Geometry check sheet. Reference: the model listing, model coordinates, mm. Face numbers are marked on the shaded views. A direction names the side the tool comes from. Round coordinates to 2 decimals unless told otherwise and drop trailing zeros. Loops run counter-clockwise (first coordinate to the right, second up) from the corner with the lowest first, then second, coordinate; pieces in that order, holes last.
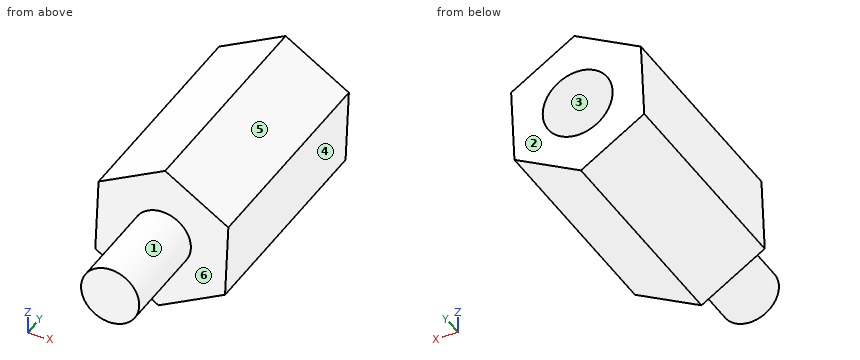
```python
from build123d import *

# Parameters (mm, degrees)
BOSS_EXTRUDE1_DEPTH = 11.1125
SKETCH2_R           = 1.4224
BOSS_EXTRUDE2_DEPTH = 4.7625
SKETCH3_R           = 1.70891155
CUT_EXTRUDE1_DEPTH  = 6.35


with BuildPart() as part:
    # Sketch1 → Boss-Extrude1 (new body)
    with BuildSketch(Plane(origin=(0, 0, 0), x_dir=(1, 0, 0), z_dir=(0, 1, 0))):
        Polygon((3.252691355, -1.691399504), (3.091140616, 1.971213592), (-0.161550739, 3.662613096), (-3.252691355, 1.691399504), (-3.091140616, -1.971213592), (0.161550739, -3.662613096), align=None)
    extrude(amount=BOSS_EXTRUDE1_DEPTH)

    # Sketch2 → Boss-Extrude2 (add)
    with BuildSketch(Plane.XZ):
        Circle(SKETCH2_R)
    extrude(amount=BOSS_EXTRUDE2_DEPTH)

    # Sketch3 → Cut-Extrude1 (cut)
    with BuildSketch(Plane(origin=(0, 11.1125, 0), x_dir=(1, 0, 0), z_dir=(0, 1, 0))):
        Circle(SKETCH3_R)
    extrude(amount=-CUT_EXTRUDE1_DEPTH, mode=Mode.SUBTRACT)


solid = part.part
```
1) Mould release check, pull along Z, two halves, no side actions. Record for the marked faces 3, 4, 5 and 6: +Z half, -Z half, draft (parallel to the pull), parting line (faces both ways), or undercut.
Report:
face 3: undercut
face 4: -Z half
face 5: +Z half
face 6: draft
2) Gauge pin test, flat ends, axial feed: pin 1 (1 mm diameter, centred on x = -1.5, y = 2, fed in from +Z); pin 2 (4 mm diameter, centred on y = 0.5, z = 0.5, fed in from -X); pin 3 (1.5 mm diameter, centred on y = 2.5, z = 0.5, fed in from +X). Record the tip position at first contact, or that the pin passes through.
Report:
pin 1: stops at z = 3.06
pin 2: stops at x = -3.24
pin 3: stops at x = 3.23
3) Sectioned sample at A-A, the plane y = 6. Record the cut outline in (x, z), then the cut area to 3 significant figures.
Report:
outline: (-3.25, -1.69) - (-0.16, -3.66) - (3.09, -1.97) - (3.25, 1.69) - (0.16, 3.66) - (-3.09, 1.97) - close; hole circle Ø3.42 at (0, 0)
area: 25.7 mm2
4) Sectioned sample at C-C, the plane x = 1.25. Record the cut outline in (y, z), then the cut area to 3 significant figures.
Report:
outline: (-4.76, -0.68) - (0, -0.68) - (0, -2.93) - (11.11, -2.93) - (11.11, -1.17) - (4.76, -1.17) - (4.76, 1.17) - (11.11, 1.17) - (11.11, 2.97) - (0, 2.97) - (0, 0.68) - (-4.76, 0.68) - close
area: 57.2 mm2
5) Sectioned sample at B-B, the plane z = 0. Record the cut outline in (x, y), then the cut area to 3 significant figures.
Report:
outline: (-3.18, 0) - (-1.42, 0) - (-1.42, -4.76) - (1.42, -4.76) - (1.42, 0) - (3.18, 0) - (3.18, 11.11) - (1.71, 11.11) - (1.71, 4.76) - (-1.71, 4.76) - (-1.71, 11.11) - (-3.18, 11.11) - close
area: 62.5 mm2
6) Scan lines: line 1 along Y through (x, z) = (-0.25, 0); line 2 along Z through (x, y) = (0, 7.25); line 3 along Y through (x, z) = (-2.75, 1). Record each from-to range of solid material in increasing order.
Report:
line 1: y = -4.76 to 4.76
line 2: z = -3.58 to -1.71, 1.71 to 3.58
line 3: y = 0 to 11.11
7) Access from +Z, -Z, +X, -X, +Y, -Y to the whole of each face (thin tool, end or side, straight path). Record for the marked faces 1 and 2.
Report:
face 1: -Y
face 2: +Z, -Z, +X, -X, +Y
8) Sectioned sample at D-D, the plane y = 3. Record the cut outline in (x, z), then the cut area to 3 significant figures.
Report:
outline: (-3.25, -1.69) - (-0.16, -3.66) - (3.09, -1.97) - (3.25, 1.69) - (0.16, 3.66) - (-3.09, 1.97) - close
area: 34.9 mm2
